Job drawing, mm, ordinate dimensions from the low corner. One solid piece. Give positions to 0.01 mm unless a question says otherwise; leave off trailing zeros. Write each loop counter-clockwise with the first axis right and the second up, starting at its lowest first coordinate (ties: lowest second). Pieces come first, ordered by that corner, then holes. Notation, with made-up numbers: M 29.25,25 L 73.25,25 A35 cw 73.25,63 Z; hole C 61.25,69 d10. An arc over 180 degrees is marked long. Answer as CSV lines item,"result". Start each with the question number.
Item 1: Band-saw the part on B-B, the plane y = 0.85. List the corners of the cut face in (x, z).
Item 2: Wall check: L1, parallel to X at y = 2.8, z = 105.5; L2, parallel to Z at x = 218.5, y = 0.4. Give the ranges that are in metal, low to high. Write a range as from..to.
Item 3: Band-saw the part on C-C, the plane x = 89.5. List the corners of the cut face in (y, z) (1 decimal), then the cut area to 3 significant figures.
Item 4: Pin check, flat tip, straight feed: pin 1 (1 mm diameter, centred on y = 1.5, z = 123.5, fed in from -X). Stop position of the tip, or through.
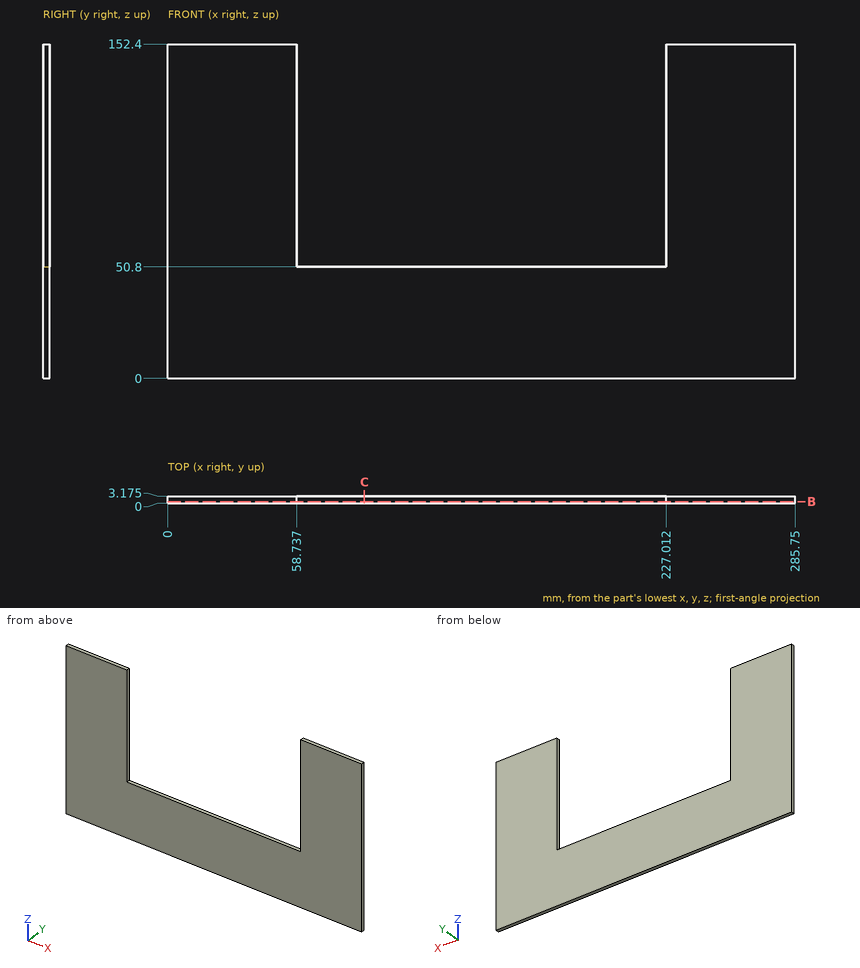
Output:
1,outline,"M 0,0 L 285.75,0 L 285.75,152.4 L 227.01,152.4 L 227.01,50.8 L 58.74,50.8 L 58.74,152.4 L 0,152.4 Z"
2,L1,"0..58.74, 227.01..285.75"
2,L2,"0..50.8"
3,outline,"M 0,0 L 3.2,0 L 3.2,50.8 L 0,50.8 Z"
3,area,"161 mm²"
4,pin 1,"x = 0"
